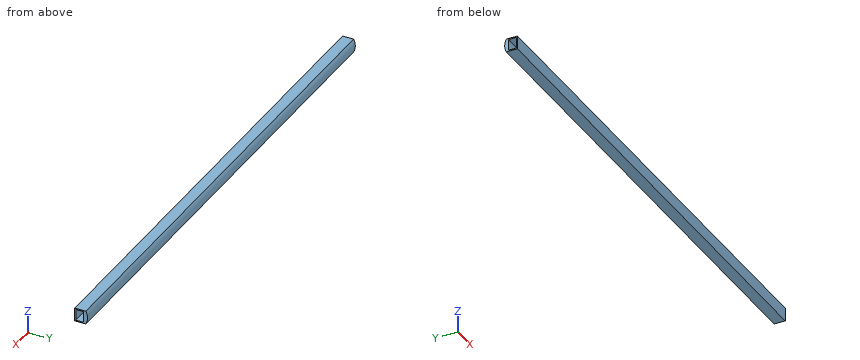
```python
from build123d import *

# Parameters (mm, degrees)
CROQUIS1_W              = 460
CROQUIS1_H              = 12
SALIENTE_EXTRUIR1_DEPTH = 10
CROQUIS2_W              = 10
CROQUIS2_H              = 7
CORTAR_EXTRUIR1_DEPTH   = 970
SALIENTE_EXTRUIR2_DEPTH = 460


with BuildPart() as part:
    # Croquis1 → Saliente-Extruir1 (new body)
    with BuildSketch(Plane(origin=(0, 0, 0), x_dir=(1, 0, 0), z_dir=(0, 1, 0))):
        with Locations((230, 6)):
            Rectangle(CROQUIS1_W, CROQUIS1_H)
    extrude(amount=SALIENTE_EXTRUIR1_DEPTH)

    # Croquis2 → Cortar-Extruir1 (cut)
    with BuildSketch(Plane.ZY):
        with Locations((-6, 4.5)):
            Rectangle(CROQUIS2_W, CROQUIS2_H)
    extrude(amount=-CORTAR_EXTRUIR1_DEPTH, mode=Mode.SUBTRACT)

    # Croquis3 → Saliente-Extruir2 (add)
    with BuildSketch(Plane.ZY):
        with BuildLine():
            ThreePointArc((0, 10), (-6, 11.465101961), (-12, 10))
            Line((-12, 10), (0, 10))
        make_face()
    extrude(amount=-SALIENTE_EXTRUIR2_DEPTH)


solid = part.part
```
Design review of the part built by this model. Coordinates are the model's own, in mm. Round coordinates to 2 decimals unless told otherwise and drop trailing zeros. Order: outer loops, then holes, each group sorted by start corner. A loop starts at its lowest first (then second) coordinate and runs counter-clockwise, first axis right, second up. Notation, with made-up numbers: (76, 82) - (93, 82) arc R24 ccw to (93, 97) - close; hole circle Ø3 at (54.5, 10). An arc over 180 degrees is marked (long way). Return JSON: item names as keys, results as strings.
Q1. Wall thickness on L1, parallel to Z at x = 313, y = 7; L2, parallel to Y at x = 81.5, z = -4.5; L3, parallel to Y at x = 324, z = -9.5: over which ranges is each line inside the solid? List them lowest first. Write a range as [from, to].
Computed values:
{"L1": "z = [-12, -11], [-1, 0]", "L2": "y = [0, 1], [8, 11.38]", "L3": "y = [0, 1], [8, 10.99]"}
Q2. Consider section C-C on z = -7.25. Write out the cut boundary in (x, y).
Computed values:
{"outline": "(0, 0) - (460, 0) - (460, 1) - (0, 1) - close; (0, 8) - (460, 8) - (460, 11.4) - (0, 11.4) - close"}
Q3. Consider section A-A on y = 6. Write out the cut boundary in (x, z).
Computed values:
{"outline": "(0, -12) - (460, -12) - (460, -11) - (0, -11) - close; (0, -1) - (460, -1) - (460, 0) - (0, 0) - close"}
Q4. Consider section B-B on x = 138.5. Write out the cut boundary in (y, z).
Computed values:
{"outline": "(0, -12) - (10, -12) arc R13.02 ccw to (10, 0) - (0, 0) - close; hole (1, -11) - (8, -11) - (8, -1) - (1, -1) - close"}
Q5. For pin 1 Ø1.5 at (y, z) = (8.5, -6.5) entering from -X, flat-tipped, find the tip position at first contact; note if it passes through.
Computed values:
{"pin 1": "stops at x = 0"}
